Build history of the part. All positions in model axes, mm. A direction names the side the tool comes from. Round coordinates to 2 decimals unless told otherwise and drop trailing zeros. Order: outer loops, then holes, each group sorted by start corner. A loop starts at its lowest first (then second) coordinate and runs counter-clockwise, first axis right, second up. Notation, with made-up numbers: (30, 27.25) -> (82, 27.25) arc R20 cw to (82, 39.25) -> close; hole circle Ø7 at (-27.5, 66.5). An arc over 180 degrees is marked (long way). Write item = value, one per line.
from build123d import *

# Parameters (mm, degrees)
F1_DEPTH  = 50
F2_T      = -2
F3_R      = 2.5
F3_R_2    = 1.25
F4_DEPTH  = 30
F5_W      = 9
F5_H      = 5
F6_DEPTH  = 2
F8_R      = 4.25
F8_W      = 13
F8_H      = 20
F9_DEPTH  = 2
F10_R     = 2.5
F10_R_2   = 1.25
F11_DEPTH = 5
F12_R     = 3.8125
F13_DEPTH = 25


with BuildPart() as f1:
    # F0 (on Top) → F1 (new body)
    with BuildSketch(Plane.XY):
        with BuildLine():
            Line((70, 65), (-70, 65))
            ThreePointArc((-70, 65), (-80.606602, 60.606602), (-85, 50))
            Line((-85, 50), (-85, -50))
            ThreePointArc((-85, -50), (-80.606602, -60.606602), (-70, -65))
            Line((-70, -65), (70, -65))
            ThreePointArc((70, -65), (80.606602, -60.606602), (85, -50))
            Line((85, -50), (85, 50))
            ThreePointArc((85, 50), (80.606602, 60.606602), (70, 65))
        make_face()
    extrude(amount=F1_DEPTH)

    # F2
    f2_openings = [f1.faces().sort_by_distance(p)[0] for p in [
        (0, 0, 50),
    ]]
    offset(amount=F2_T, openings=f2_openings)

    # F3 (on face) → F4 (join)
    with BuildSketch(Plane.XY.offset(2)):
        with Locations((3.175, 59.825)):
            Circle(F3_R)
        with Locations((3.175, 59.825)):
            Circle(F3_R_2, mode=Mode.SUBTRACT)
        with Locations((3.175, 16.175)):
            Circle(F3_R)
        with Locations((3.175, 16.175)):
            Circle(F3_R_2, mode=Mode.SUBTRACT)
        with Locations((66.825, 59.825)):
            Circle(F3_R)
        with Locations((66.825, 59.825)):
            Circle(F3_R_2, mode=Mode.SUBTRACT)
        with Locations((66.825, 16.175)):
            Circle(F3_R)
        with Locations((66.825, 16.175)):
            Circle(F3_R_2, mode=Mode.SUBTRACT)
    extrude(amount=F4_DEPTH)

    # F5 (on face) → F6 (cut, through all)
    with BuildSketch(Plane(origin=(0, 65, 0), x_dir=(-1, 0, 0), z_dir=(0, 1, 0))):
        with Locations((-16, 39)):
            Rectangle(F5_W, F5_H)
    extrude(amount=-F6_DEPTH, mode=Mode.SUBTRACT)

    # F8 (on face) → F9 (cut, through all)
    with BuildSketch(Plane.YZ.offset(85)):
        with Locations((17.588826, 25)):
            Circle(F8_R)
        with Locations((37.588826, 25)):
            Rectangle(F8_W, F8_H)
    extrude(amount=-F9_DEPTH, mode=Mode.SUBTRACT)

    # F10 (on face) → F11 (join)
    with BuildSketch(Plane.XY.offset(2)):
        with Locations((66.973306, 0)):
            Circle(F10_R)
        with Locations((66.973306, 0)):
            Circle(F10_R_2, mode=Mode.SUBTRACT)
    extrude(amount=F11_DEPTH)

    # F12 (on face) → F13 (cut)
    with BuildSketch(Plane.YZ.offset(85)):
        with Locations((-30, 10)):
            Circle(F12_R)
    extrude(amount=-F13_DEPTH, mode=Mode.SUBTRACT)


solid = f1.part
Q1. Cut at A-A, the plane y = -30. List the corners of the cut face in (x, z).
Check values:
outline = (-85, 0) -> (85, 0) -> (85, 6.19) -> (83, 6.19) -> (83, 2) -> (-83, 2) -> (-83, 50) -> (-85, 50) -> close; (83, 13.81) -> (85, 13.81) -> (85, 50) -> (83, 50) -> close
Q2. Mould opens along X. For faces 1 (the face through (79.091, -59.293, 25.664)), 2 (the face through (4, 61, 32)), 3 (the face through (80.72, 60.49, 24.65)), 4 (the face through (-1, 1, 0)) say: released by +X, released by -X, zero draft, split by the parting line, or undercut.
Check values:
face_1 = undercut
face_2 = undercut
face_3 = released by +X
face_4 = zero draft
Q3. Which spindle directions (+Z, -Z, +X, -X, +Y, -Y) get a long thin tool onto all of the face, cutting with end or side? Do faces 5 (the face through (1, 63, 26)), 6 (the face through (85, -1, 25)), 7 (the face through (84.01, -26.48, 8.54)). Say none if no direction does.
Check values:
face_5 = +Z
face_6 = +Z, -Z, +X, +Y, -Y
face_7 = +X
Q4. Cut at B-B, the plane z = 10. Give the number of separate pieces and of enclosed holes in the cut face, and give its area (3 significant figures).
Check values:
separate_pieces = 5
enclosed_holes = 4
area = 1,180 mm²
Q5. Probe probe 1 along Y at (x, z) = (-15, 7); probe 2 along X at (y, z) = (-24, 40); probe 3 along Z at (x, y) = (84, -30). List the from-to ranges inside material, lowest first.
Check values:
probe_1 = -65 to -63, 63 to 65
probe_2 = -85 to -83, 83 to 85
probe_3 = 0 to 6.19, 13.81 to 50
Q6. Cut at D-D, the plane x = -21. List the corners of the cut face in (y, z), and give its area (3 significant figures).
Check values:
outline = (-65, 0) -> (65, 0) -> (65, 50) -> (63, 50) -> (63, 2) -> (-63, 2) -> (-63, 50) -> (-65, 50) -> close
area = 452 mm²
Q7. Flat gauge pins, fed straight in: pin 1 (8 mm diameter, centred on x = -46.5, y = 41.5, fed in from +Z); pin 2 (5.5 mm diameter, centred on x = 67.5, y = 58.5, fed in from +Z); pin 3 (0.6 mm diameter, centred on x = 83.5, z = 21, fed in from -Y). Where does each tip first touch, or does it go through?
Check values:
pin_1 = 2
pin_2 = 32
pin_3 = -57.12
